```python
from build123d import *

# Parameters (mm, degrees)
SKETCH1_W           = 10
SKETCH1_H           = 2.5
BOSS_EXTRUDE1_DEPTH = 2.5


with BuildPart() as part:
    # Sketch1 → Boss-Extrude1 (new body)
    with BuildSketch(Plane.XY):
        Polygon((65, -13.75), (60, -13.75), (60, -18.75), (50, -18.75), (50, -13.75), (40, -13.75), (40, -18.75), (30, -18.75), (30, -13.75), (20, -13.75), (20, -18.75), (10, -18.75), (10, -13.75), (-10, -13.75), (-10, -18.75), (-20, -18.75), (-20, -13.75), (-30, -13.75), (-30, -18.75), (-40, -18.75), (-40, -13.75), (-50, -13.75), (-50, -18.75), (-60, -18.75), (-60, -13.75), (-65, -13.75), (-65, 16.25), (-60, 16.25), (-60, 18.75), (-50, 18.75), (-50, 16.25), (-40, 16.25), (-40, 18.75), (-30, 18.75), (-30, 16.25), (-20, 16.25), (-20, 18.75), (-10, 18.75), (-10, 16.25), (10, 16.25), (10, 18.75), (20, 18.75), (20, 16.25), (30, 16.25), (30, 18.75), (40, 18.75), (40, 16.25), (50, 16.25), (50, 18.75), (60, 18.75), (60, 16.25), (65, 16.25), align=None)
        with Locations((-15, -7.5)):
            Rectangle(SKETCH1_W, SKETCH1_H, mode=Mode.SUBTRACT)
        with Locations((-35, -7.5)):
            Rectangle(SKETCH1_W, SKETCH1_H, mode=Mode.SUBTRACT)
        with Locations((15, -7.5)):
            Rectangle(SKETCH1_W, SKETCH1_H, mode=Mode.SUBTRACT)
        with Locations((35, -7.5)):
            Rectangle(SKETCH1_W, SKETCH1_H, mode=Mode.SUBTRACT)
    extrude(amount=BOSS_EXTRUDE1_DEPTH)


solid = part.part
```
Here's how the part is built. I have some questions about the finished solid (model axes, mm). A direction names the side the tool comes from. Round coordinates to 2 decimals unless told otherwise and drop trailing zeros. Write each loop counter-clockwise with the first axis right and the second up, starting at its lowest first coordinate (ties: lowest second). Pieces come first, ordered by that corner, then holes.
Q1. If we section it at A-A on y = -15.5: Write out the boundary of the cut face in (x, z), plus the area to 3 significant figures.
Q2. If we mould it in two halves opening along X, with no side actions, what happens to faces 5 (the flat face through (55, -18.75, 1)), 6 (the flat face through (-40, -16, 1))? For each: +X half, -X half, draft (parallel to the pull), parting line (faces both ways), or undercut.
Q3. Which directions (+Z, -Z, +X, -X, +Y, -Y) give clear straight access to the entire face, cutting with the end or side of a thin tool? Please do faces 1 (the flat face through (-62, -13.75, 1)), 2 (the flat face through (-25, -13.75, 1)), 3 (the flat face through (-15, -8.75, 1)), 4 (the flat face through (-40, 17, 1)).
Q4. If we section it at D-D on x = 23.5: Write out the boundary of the cut face in (y, z), plus the area to 3 significant figures.
Q5. If we section it at B-B on x = -36: Write out the boundary of the cut face in (y, z).
Q6. If we section it at C-C on z = 0.95: Give the number of separate pieces and of enclosed holes in the cut face, plus the area to 3 significant figures.
Q7. Will these pins go through, and if not, where does the flat tip stop? P1, Ø1.2, axis at x = 3.5, z = 1.5, coming from the -Y side; P2, Ø0.8, axis at y = 18, z = 1, coming from the -X side; P3, Ø1.5, axis at x = 29, z = 0.5, coming from the +Y side.
Q8. Please list where these lines run through material, in increasing order: probe 1 along X at (y, z) = (-15, 1.8); probe 2 along X at (y, z) = (-8.5, 0.5); probe 3 along Y at (x, z) = (-34, 0.8).
Answer below:
1. outline: (-60, 0) - (-50, 0) - (-50, 2.5) - (-60, 2.5) - close; (-40, 0) - (-30, 0) - (-30, 2.5) - (-40, 2.5) - close; (-20, 0) - (-10, 0) - (-10, 2.5) - (-20, 2.5) - close; (10, 0) - (20, 0) - (20, 2.5) - (10, 2.5) - close; (30, 0) - (40, 0) - (40, 2.5) - (30, 2.5) - close; (50, 0) - (60, 0) - (60, 2.5) - (50, 2.5) - close
1. area: 150 mm2
2. face 5: draft
2. face 6: undercut
3. face 1: +Z, -Z, -X, -Y
3. face 2: +Z, -Z, -Y
3. face 3: +Z, -Z
3. face 4: +Z, -Z, +Y
4. outline: (-13.75, 0) - (16.25, 0) - (16.25, 2.5) - (-13.75, 2.5) - close
4. area: 75.0 mm2
5. outline: (-18.75, 0) - (-8.75, 0) - (-8.75, 2.5) - (-18.75, 2.5) - close; (-6.25, 0) - (18.75, 0) - (18.75, 2.5) - (-6.25, 2.5) - close
6. separate pieces: 1
6. enclosed holes: 4
6. area: 4,250 mm2
7. P1: stops at y = -13.75
7. P2: stops at x = -60
7. P3: stops at y = 16.25
8. probe 1: x = -60 to -50, -40 to -30, -20 to -10, 10 to 20, 30 to 40, 50 to 60
8. probe 2: x = -65 to -40, -30 to -20, -10 to 10, 20 to 30, 40 to 65
8. probe 3: y = -18.75 to -8.75, -6.25 to 18.75
